from build123d import *

# Parameters (mm, degrees)
SKETCH1_W           = 80
SKETCH1_H           = 58
BOSS_EXTRUDE1_DEPTH = 3.5
BOSS_EXTRUDE2_DEPTH = 5


with BuildPart() as part:
    # Sketch1 → Boss-Extrude1 (new body)
    with BuildSketch(Plane(origin=(0, 0, 0), x_dir=(1, 0, 0), z_dir=(0, 1, 0))):
        with Locations((40, 29)):
            Rectangle(SKETCH1_W, SKETCH1_H)
    extrude(amount=BOSS_EXTRUDE1_DEPTH)

    # Sketch2 → Boss-Extrude2 (add)
    with BuildSketch(Plane(origin=(0, 0, -58), x_dir=(-1, 0, 0), z_dir=(0, 0, -1))):
        Polygon((-68, 3.5), (-80, 3.5), (-80, 0), (0, 0), (0, 3.5), (-12, 3.5), (-12, 10), (-24, 10), (-24, 3.5), (-56, 3.5), (-56, 10), (-68, 10), align=None)
    extrude(amount=BOSS_EXTRUDE2_DEPTH)


solid = part.part
Verification items for the finished model (mm, model axes). A direction names the side the tool comes from. Round coordinates to 2 decimals unless told otherwise and drop trailing zeros. Write each loop counter-clockwise with the first axis right and the second up, starting at its lowest first coordinate (ties: lowest second). Pieces come first, ordered by that corner, then holes.
(1) Material ranges on line 1 (Y direction, x = 15.5, z = -15); line 2 (Z direction, x = 13.5, y = 9), recorded low to high.
Returned:
line 1: y = 0 to 3.5
line 2: z = -63 to -58
(2) Mould release check, pull along X, two halves, no side actions. Record for faces 1 (the flat face through (0, 2, -31)), 2 (the flat face through (39, 2, 0)), 3 (the flat face through (24, 7, -60)): pulls with the +X half, pulls with the -X half, needs draft (parallel to the pull), parting line crosses it, or undercut.
Returned:
face 1: pulls with the -X half
face 2: needs draft
face 3: undercut
(3) Depth check by flat-ended pin: pin 1 Ø2.5 at (y, z) = (7, -61) entering from +X; pin 2 Ø2.5 at (y, z) = (6.5, -61.5) entering from -X; pin 3 Ø1.5 at (x, y) = (36.5, 6) entering from -Z; pin 4 Ø3 at (x, y) = (62.5, 6) entering from +Z. Enter the tip coordinate at first touch or a pass-through.
Returned:
pin 1: stops at x = 68
pin 2: stops at x = 12
pin 3: passes through
pin 4: stops at z = -58
(4) Access from +Z, -Z, +X, -X, +Y, -Y to the whole of each face (thin tool, end or side, straight path). Record for faces 4 (the flat face through (18, 7, -58)), 5 (the flat face through (68, 7, -60)), 6 (the flat face through (56, 7, -60)), 7 (the flat face through (12, 7, -60)).
Returned:
face 4: +Z, +X, -X, +Y
face 5: +Z, -Z, +X, +Y
face 6: +Z, -Z, +Y
face 7: +Z, -Z, -X, +Y
(5) Section check D-D (x = 20). Enter the section's corners in (y, z).
Returned:
outline: (0, -63) - (10, -63) - (10, -58) - (3.5, -58) - (3.5, 0) - (0, 0) - close
(6) Section check A-A (y = 5). Enter the section's corners in (x, z), plus the area to 3 significant figures.
Returned:
outline: (12, -63) - (24, -63) - (24, -58) - (12, -58) - close; (56, -63) - (68, -63) - (68, -58) - (56, -58) - close
area: 120 mm2
(7) Section check C-C (z = -8). Enter the section's corners in (x, y).
Returned:
outline: (0, 0) - (80, 0) - (80, 3.5) - (0, 3.5) - close
(8) Section check B-B (x = 47.5). Enter the section's corners in (y, z).
Returned:
outline: (0, -63) - (3.5, -63) - (3.5, 0) - (0, 0) - close
